Autodesk Inventor part; units mm, degrees
ref_plane "YZ Plane" through (0, 0, 0) normal (1, 0, 0) x (0, 1, 0)
ref_plane "XZ Plane" through (0, 0, 0) normal (0, 1, 0) x (-1, 0, 0)
ref_plane "XY Plane" through (0, 0, 0) normal (0, 0, 1) x (1, 0, 0)
sketch "Sketch1" plane through (0, 0, 0) normal (0, 1, 0) x (-1, 0, 0)
  line L0 (-12.7, 25.4) -> (12.7, 25.4)
  line L1 (12.7, 25.4) -> (12.7, -25.4)
  line L2 (12.7, -25.4) -> (-12.7, -25.4)
  line L3 (-12.7, -25.4) -> (-12.7, 25.4)
  line L4 (-12.7, 25.4) -> (12.7, -25.4) construction
  line L5 (12.7, 25.4) -> (-12.7, -25.4) construction
  point P0 (0, 0)
  dimension "d0" = 50.8
  dimension "d1" = 25.4
extrude "Extrusion1" add sketch "Sketch1" along normal blind 127
shell "Shell1" thickness 3.175 removed faces 2 at (-4.2333, 0, 8.4667) at (-4.2333, 127, 8.4667)
sketch "Sketch2" plane through (-12.7, 0, -25.4) normal (-1, 0, 0) x (0, 0, 1)
  line L0 (9.9, 90.5) -> (40.9, 90.5)
  line L1 (40.9, 90.5) -> (40.9, 121.5)
  line L2 (40.9, 121.5) -> (9.9, 121.5)
  line L3 (9.9, 121.5) -> (9.9, 90.5)
  line L4 (9.9, 90.5) -> (40.9, 121.5) construction
  line L5 (40.9, 90.5) -> (9.9, 121.5) construction
  line L6 (0, 127) -> (50.8, 127)
  point P0 (25.4, 0)
  point P1 (25.4, 106)
  point P2 (25.4, 106)
  point P3 (25.4, 127)
  dimension "d5" = 31
  dimension "d6" = 31
  dimension "d7" = 21
hole "Hole1" at (-12.7, 121.5, -15.5) at (-12.7, 121.5, 15.5) at (-12.7, 90.5, 15.5) at (-12.7, 90.5, -15.5) direction (1, 0, 0) diameter 3.2 end through all counterbore diameter 7.5 counterbore depth 5
hole "Hole2" at (-12.7, 106, 0) direction (1, 0, 0) diameter 10 end through all
sketch "Sketch3" plane through (12.7, 0, 25.4) normal (1, 0, 0) x (0, 0, -1)
  circle A0 centre (25.4, 106) radius 5
  circle A1 centre (25.4, 106) radius 11.5
  point P0 (25.4, 0)
  dimension "d22" = 23
extrude "Extrusion2" cut sketch "Sketch3" against normal up to surface (22.225 mm away) contours A0 | A1
sketch "Sketch4" plane through (12.7, 0, 25.4) normal (1, 0, 0) x (0, 0, -1)
  circle A0 centre (25.4, 18) radius 8
  line L0 (50.8, 0) -> (0, 0)
  point P0 (25.4, 0)
  point P1 (25.4, 0)
  dimension "d25" = 16
  dimension "d26" = 18
extrude "Extrusion3" cut sketch "Sketch4" against normal through all
sketch "Sketch6" plane through (12.7, 0, -25.4) normal (0, 0, -1) x (-1, 0, 0)
  line L0 (12.7, 63.5) -> (12.7, 114.3)
  line L1 (25.4, 0) -> (0, 0)
  line L2 (0, 127) -> (25.4, 127)
  line L3 (25.4, 0) -> (25.4, 127)
  point P0 (12.7, 0)
  point P1 (12.7, 88.9)
  point P2 (12.7, 0)
  dimension "d55" = 50.8
  dimension "d61" = 38.1
hole "Hole4" at (0, 88.9, -25.4) at (0, 114.3, -25.4) at (0, 63.5, -25.4) direction (0, 0, 1) diameter 3.242 end through all
sketch "Sketch7" plane through (12.7, 0, 25.4) normal (1, 0, 0) x (0, 0, -1)
  circle A0 centre (25.4, 18) radius 8
  line L0 (7.4, 18) -> (43.4, 18)
  point P0 (25.4, 0)
  dimension "d47" = 36
hole "Hole5" at (12.7, 18, -18) at (12.7, 18, 18) direction (-1, 0, 0) diameter 3.242 end through all
pattern_linear "Rectangular Pattern1" count 2 spacing 50.8 along (0, -1, 0) of "Hole4"
equation "\"d6\" = d5"
properties part number "Transmission_Case_Long"
Check sheet for the modelled part. Datum: model origin and axes. Units: mm. A direction names the side the tool comes from. Round coordinates to 2 decimals unless told otherwise and drop trailing zeros. Loops run counter-clockwise (first coordinate to the right, second up) from the corner with the lowest first, then second, coordinate; pieces in that order, holes last. Notation, with made-up numbers: (77, 55) - (105, 55) arc R16 ccw to (105, 66) - close; hole circle Ø10 at (78, 1). An arc over 180 degrees is marked (long way). Write item = value, one per line. Start each with the question number.
Q1. Depth check by flat-ended pin: P1, Ø5, axis at y = 121.5, z = -15.5, coming from the -X side (3 decimals). Enter the tip coordinate at first touch or a pass-through.
Q2. Section check D-D (z = 21). Record the boundary of the cut face in (x, y) (3 decimals), plus the area to 3 significant figures.
Q3. Thickness scan on L1, parallel to Y at x = 11.9, z = 0; L2, parallel to Y at x = 0, z = 23; L3, parallel to Y at x = -10.55, z = -15.5. Record the ranges inside material, lowest first.
Q4. Section check B-B (z = 0). Record the boundary of the cut face in (x, y) (3 decimals).
Q5. Release check for a two-part mould opening along Y. For faces 4 (the face through (10, 127, -2)), 5 (the face through (0.621, 14.197, 23.835)), 6 (the face through (2, 63, -22.225)) record: pulls with the +Y half, pulls with the -Y half, needs draft (parallel to the pull), parting line crosses it, or undercut.
Q6. Section check C-C (y = 63.5). Record the boundary of the cut face in (x, z) (3 decimals).
Q7. Access from +Z, -Z, +X, -X, +Y, -Y to the whole of each face (thin tool, end or side, straight path). Record for faces 1 (the face through (-11.09, 117.782, -15.988)), 2 (the face through (-2, 63, 22.225)), 3 (the face through (-3, 63, 25.4)).
Q8. Section check A-A (y = 18). Count the separate pieces of the cut face and the enclosed holes in it, plus the area to 3 significant figures.
Derived:
q1.P1 = 9.525
q2.outline = (-12.7, 0) - (-9.525, 0) - (-9.525, 127) - (-12.7, 127) - close; (9.525, 0) - (12.7, 0) - (12.7, 127) - (9.525, 127) - close
q2.area = 806 mm^2
q3.L1 = 0 to 10, 26 to 94.5, 117.5 to 127
q3.L2 = 0 to 11.08, 14.32 to 36.48, 39.72 to 61.88, 65.12 to 87.28, 90.52 to 112.68, 115.92 to 127
q3.L3 = 0 to 86.75, 94.25 to 117.75, 125.25 to 127
q4.outline = (-12.7, 0) - (-9.525, 0) - (-9.525, 10) - (-12.7, 10) - close; (-12.7, 26) - (-9.525, 26) - (-9.525, 101) - (-12.7, 101) - close; (-12.7, 111) - (-9.525, 111) - (-9.525, 127) - (-12.7, 127) - close; (9.525, 0) - (12.7, 0) - (12.7, 10) - (9.525, 10) - close; (9.525, 26) - (12.7, 26) - (12.7, 94.5) - (9.525, 94.5) - close; (9.525, 117.5) - (12.7, 117.5) - (12.7, 127) - (9.525, 127) - close
q5.face_4 = pulls with the +Y half
q5.face_5 = undercut
q5.face_6 = needs draft
q6.outline = (-12.7, -25.4) - (-1.621, -25.4) - (-1.621, -22.225) - (-9.525, -22.225) - (-9.525, 22.225) - (-1.621, 22.225) - (-1.621, 25.4) - (-12.7, 25.4) - close; (1.621, -25.4) - (12.7, -25.4) - (12.7, 25.4) - (1.621, 25.4) - (1.621, 22.225) - (9.525, 22.225) - (9.525, -22.225) - (1.621, -22.225) - close
q7.face_1 = -X
q7.face_2 = +Y, -Y
q7.face_3 = +Z, +X, -X, +Y, -Y
q8.separate_pieces = 6
q8.enclosed_holes = 0
q8.area = 301 mm^2
